Autodesk Inventor part; units mm, degrees
ref_plane "YZ Plane" through (0, 0, 0) normal (1, 0, 0) x (0, 1, 0)
ref_plane "XZ Plane" through (0, 0, 0) normal (0, 1, 0) x (-1, 0, 0)
ref_plane "XY Plane" through (0, 0, 0) normal (0, 0, 1) x (1, 0, 0)
sketch "Sketch1" plane through (0, 0, 0) normal (0, 1, 0) x (-1, 0, 0)
  circle A0 centre (0, 0) radius 4.425
  line L0 (-11.1809, -4.4215) -> (-11.6444, -2.9949)
  line L1 (-11.6444, -2.9949) -> (-6.3005, -1.2586)
  arc A1 (-4.3575, 4.7216) -> (-6.3005, -1.2586) centre (0, 0) ccw
  line L2 (-4.3575, 4.7216) -> (-7.6602, 9.2674)
  line L3 (-7.6602, 9.2674) -> (-6.4467, 10.149)
  line L4 (-6.4467, 10.149) -> (-3.1439, 5.6032)
  arc A2 (3.1439, 5.6032) -> (-3.1439, 5.6032) centre (0, 0) ccw
  line L5 (3.1439, 5.6032) -> (6.4467, 10.149)
  line L6 (6.4467, 10.149) -> (7.6602, 9.2674)
  line L7 (7.6602, 9.2674) -> (4.3575, 4.7216)
  arc A3 (6.3005, -1.2586) -> (4.3575, 4.7216) centre (0, 0) ccw
  line L8 (6.3005, -1.2586) -> (11.6444, -2.9949)
  line L9 (11.6444, -2.9949) -> (11.1809, -4.4215)
  line L10 (11.1809, -4.4215) -> (5.837, -2.6852)
  arc A4 (0.75, -6.3811) -> (5.837, -2.6852) centre (0, 0) ccw
  line L11 (0.75, -6.3811) -> (0.75, -12)
  line L12 (0.75, -12) -> (-0.75, -12)
  line L13 (-0.75, -12) -> (-0.75, -6.3811)
  arc A5 (-5.837, -2.6852) -> (-0.75, -6.3811) centre (0, 0) ccw
  line L14 (-5.837, -2.6852) -> (-11.1809, -4.4215)
extrude "Extrusion1" add sketch "Sketch1" along normal blind 21
sketch "Sketch2" plane through (0, 21, 0) normal (0, 1, 0) x (1, 0, 0)
  circle A0 centre (0, 0) radius 11.01
  circle A1 centre (0, 0) radius 19
  dimension "d2" = 38
extrude "Extrusion2" add sketch "Sketch2" along normal blind 8.5
sketch "Sketch3" plane through (0, 21, 0) normal (0, 1, 0) x (1, 0, 0)
  circle A0 centre (0, 0) radius 11.01
extrude "Extrusion3" add sketch "Sketch3" along normal blind 1.5
sketch "Sketch4" plane through (0, 21, 0) normal (0, -1, 0) x (1, 0, 0)
  circle A0 centre (0, 0) radius 19
  dimension "d7" = 38
extrude "Extrusion4" add sketch "Sketch4" along normal blind 0.5
properties part number "eje rodaje b"
Design review of the part built by this model. Coordinates are the model's own, in mm. A direction names the side the tool comes from. Coordinates: 2 decimals unless noted, no trailing zeros. Loops run counter-clockwise (first coordinate to the right, second up) from the corner with the lowest first, then second, coordinate; pieces in that order, holes last. Notation, with made-up numbers: (-5, -9) -> (41, -9) arc R30 cw to (41, 16) -> close; hole circle Ø9 at (65.25, -25). An arc over 180 degrees is marked (long way). Use a Markdown table: item, result. Add a question column.
Item 1: We need section C-C, the plane z = 0. Write out the cut boundary in (x, y) (3 decimals).
Item 2: Wall thickness on L1, parallel to X at y = 12.5, z = 0 (3 decimals); L2, parallel to Z at x = 0, y = 25.5: over which ranges is each line inside the solid? List them lowest first. Write a range as from..to.
Item 3: We need section D-D, the plane y = 26.25. Write out the cut boundary in (x, z).
Item 4: Machinability: for faces 1 (the cylindrical face through (0.046, 10.106, 6.425)), 2 (the flat face through (0.75, 10, -9)), 3 (the cylindrical face through (3.739, 10.106, -5.225)), 4 (the flat face through (0, 22.5, 0)), which of the approach directions +Z, -Z, +X, -X, +Y, -Y give a long, thin tool a straight path to every point of the face, cutting with its end or side? Answer none if there is none.
Item 5: Clearance check with flat-ended pins moving along their axes: P1, Ø8, axis at y = 4, z = -1, coming from the +X side; P2, Ø4.5, axis at x = 0, z = -0.5, coming from the -Y side; P3, Ø3, axis at y = 20, z = -14, coming from the +X side. State where each tip first meets the part, or that it passes through.
Item 6: We need section B-B, the plane x = 0. Write out the cut boundary in (y, z) (3 decimals).
Item 7: The part is to be moulded in two halves that separate along Z. For faces 5 (the flat face through (-8.546, 10.106, -3.566)), 6 (the flat face through (4.4, 0, 1.6)), 7 (the cylindrical face through (-6.096, 10.106, 2.029)), 8 (the flat face through (7.062, 10.106, 9.702)), say which applies: +Z half, -Z half, draft (parallel to the pull), parting line (faces both ways), or undercut.
Numbers:
| question | item | result |
|---|---|---|
| 1 | outline | (-19, 20.5) -> (-6.425, 20.5) -> (-6.425, 0) -> (-4.425, 0) -> (-4.425, 20.5) -> (4.425, 20.5) -> (4.425, 0) -> (6.425, 0) -> (6.425, 20.5) -> (19, 20.5) -> (19, 29.5) -> (11.01, 29.5) -> (11.01, 22.5) -> (-11.01, 22.5) -> (-11.01, 29.5) -> (-19, 29.5) -> close |
| 2 | L1 | x = -6.425..-4.425, 4.425..6.425 |
| 2 | L2 | z = -19..-11.01, 11.01..19 |
| 3 | outline | circle Ø38 at (0, 0); hole circle Ø22.02 at (0, 0) |
| 4 | face 1 | +Z, -Y |
| 4 | face 2 | -Z, +X, -Y |
| 4 | face 3 | -Z, -Y |
| 4 | face 4 | +Y |
| 5 | P1 | stops at x = 11.64 |
| 5 | P2 | stops at y = 20.5 |
| 5 | P3 | stops at x = 14.23 |
| 6 | outline | (0, -12) -> (20.5, -12) -> (20.5, -19) -> (29.5, -19) -> (29.5, -11.01) -> (22.5, -11.01) -> (22.5, 11.01) -> (29.5, 11.01) -> (29.5, 19) -> (20.5, 19) -> (20.5, 6.425) -> (0, 6.425) -> (0, 4.425) -> (20.5, 4.425) -> (20.5, -4.425) -> (0, -4.425) -> close |
| 7 | face 5 | -Z half |
| 7 | face 6 | draft |
| 7 | face 7 | undercut |
| 7 | face 8 | +Z half |
